Autodesk Inventor part; units mm, degrees
ref_plane "YZ Plane" through (0, 0, 0) normal (1, 0, 0) x (0, 1, 0)
ref_plane "XZ Plane" through (0, 0, 0) normal (0, 1, 0) x (-1, 0, 0)
ref_plane "XY Plane" through (0, 0, 0) normal (0, 0, 1) x (1, 0, 0)
sketch "Boceto4" plane through (0, 0, 0) normal (0, 0, 1) x (1, 0, 0)
  circle A0 centre (0, 140) radius 50
  circle A1 centre (150, 140) radius 25
  arc A2 (167.0429, 115.3112) -> (155, 169.5804) centre (150, 140) ccw
  arc A3 (9.1667, 194.2307) -> (-27.9698, 187.3571) centre (0, 140) ccw
  line L0 (155, 169.5804) -> (9.1667, 194.2307)
  line L1 (0, 0) -> (167.0429, 115.3112)
  line L2 (0, 0) -> (-1400, 0)
  line L3 (-27.9698, 187.3571) -> (-175.8786, 100)
  line L4 (-175.8786, 100) -> (-1300, 100)
  arc A4 (-1300, 100) -> (-1400, 0) centre (-1300, 0) ccw
  dimension "d24" = 100
  dimension "d25" = 50
  dimension "d26" = 150
  dimension "d27" = 5
  dimension "d28" = 5
  dimension "d29" = 140
  dimension "d30" = 1400
  dimension "d32" = 100
  dimension "d33" = 171.7797
extrude "Extrusión3" add sketch "Boceto4" along normal mid plane 10
sketch "Boceto5" plane through (0, 0, 0) normal (1, 0, 0) x (0, 1, 0)
  line L0 (12, -5.0363) -> (-1, -0.3047)
  line L1 (-1, -0.3047) -> (-1, -5.0363)
  line L2 (-1, -5.0363) -> (12, -5.0363)
  line L3 (12, 6.2463) -> (-1, 1.77)
  line L4 (-1, 1.77) -> (-1, 6.2463)
  line L5 (-1, 6.2463) -> (12, 6.2463)
  point P0 (0, 0)
  dimension "d36" = 1
  dimension "d37" = 13
  dimension "d38" = 13
  dimension "d39" = 70
  dimension "d40" = 71
  dimension "d41" = 0.3047
  dimension "d42" = 1.77
extrude "Extrusión4" cut sketch "Boceto5" along normal through all both and the other way through all
sketch "Boceto6" plane through (0, 0, 5) normal (0, 0, 1) x (1, 0, 0)
  circle A0 centre (150, 140) radius 25 construction
  line L0 (125, 140) -> (175, 140)
  line L1 (175, 140) -> (175, 83.3252)
  line L2 (175, 83.3252) -> (125, 83.3252)
  line L3 (125, 83.3252) -> (125, 140)
  point P0 (0, 0)
  dimension "d46" = 50
  dimension "d47" = 0
  dimension "d50" = 56.6748
extrude "Extrusión5" cut sketch "Boceto6" against normal through all
properties part number "hoja de filo"
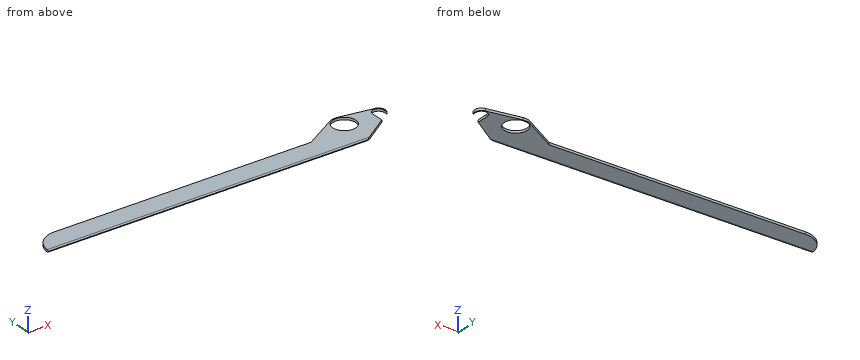
The model under review builds one solid part; all positions refer to its coordinate system, in mm. Give positions to 0.01 mm unless a question says otherwise; leave off trailing zeros. Order: outer loops, then holes, each group sorted by start corner. A loop starts at its lowest first (then second) coordinate and runs counter-clockwise, first axis right, second up. Notation, with made-up numbers: M 19.5,15.5 L 30.5,15.5 A35 cw 30.5,52.5 Z; hole C 3,5.25 d10. An arc over 180 degrees is marked long. One line per question, with ' | ' between items. Start each with the question number.
1) Consider section B-B, the plane y = 60. Give the boundary of the cut face in (x, z).
2) Wall thickness on L1, parallel to Y at x = 0, z = 1; L2, parallel to X at y = 157.5, z = -0.5; L3, parallel to Y at x = -415, z = -0.25: over which ranges is each line inside the solid? List them lowest first. Write a range as from..to.
3) Consider section A-A, the plane x = -526.5. Give the boundary of the cut face in (y, z).
4) Clearance check with flat-ended pins moving along their axes: P1, Ø3, axis at y = 156, z = -2, coming from the -X side; P2, Ø6, axis at y = 73, z = -3.5, coming from the +X side; P3, Ø4, axis at y = 86, z = -3, coming from the -X side; P4, Ø1, axis at x = -1121, z = 2, coming from the -Y side. State where each tip first meets the part, or that it passes through.
Found:
1) outline: M -1380,-5 L 86.92,-5 L 86.92,5 L -1380,5 Z
2) L1: y = 0..90, 190..195 | L2: x = -78.52..-46.84, 46.84..132.15, 167.85..174.37 | L3: y = 0..100
3) outline: M 0,-0.67 L 11.9,-5 L 100,-5 L 100,5 L 8.38,5 L 0,2.11 Z
4) P1: stops at x = -83.6 | P2: stops at x = 110.1 | P3: stops at x = -1354.26 | P4: stops at y = 0
